Input: dimensioned drawing with shaded views. Units: mm. Origin: part minimum x, y, z. A direction names the side the tool comes from. Round coordinates to 2 decimals unless told otherwise and drop trailing zeros. Loops run counter-clockwise (first coordinate to the right, second up) from the corner with the lowest first, then second, coordinate; pieces in that order, holes last.
Item 1: Section query D-D on y = 3. Return loops of the section in (x, z) (1 decimal).
Item 2: Access query for the marked faces 5, 6, 7, 8 and 9. Directions: +Z, -Z, +X, -X, +Y, -Y. A direction counts if a zero-diameter tool reaches every point of the face in a straight line with its end or side. Return the directions, or none.
Item 3: Section query B-B on z = 23.5. Return loops of the section in (x, y) (1 decimal).
Item 4: Pull-direction query (X, two-part tool) for the marked faces 1, 2, 3 and 4; classes: released by +X, released by -X, zero draft, split by the parting line, or undercut.
Item 5: Section query C-C on x = 8. Return loops of the section in (y, z) (1 decimal), then the cut area to 3 significant figures.
Item 6: Ray query, L1, parallel to X at y = 3, z = 23.75 (1 decimal); L2, parallel to X at y = 2.25, z = 6.25; L3, parallel to Y at x = 5.75, z = 12.25. Return the intervals inside material, ascending.
Item 7: Section query A-A on x = 12. Return loops of the section in (y, z) (1 decimal).
Item 8: First-contact query: P1, Ø6, axis at x = 5, z = 3, coming from the -Y side; P2, Ø3.5, axis at y = 5, z = 10.5, coming from the +X side; P3, Ø4, axis at x = 5, y = 7.5, coming from the +Z side; P4, Ø1.3, axis at x = 4.5, y = 5.5, coming from the -Z side. Flat tips, straight axial feed; report the tip coordinate or a pass-through.
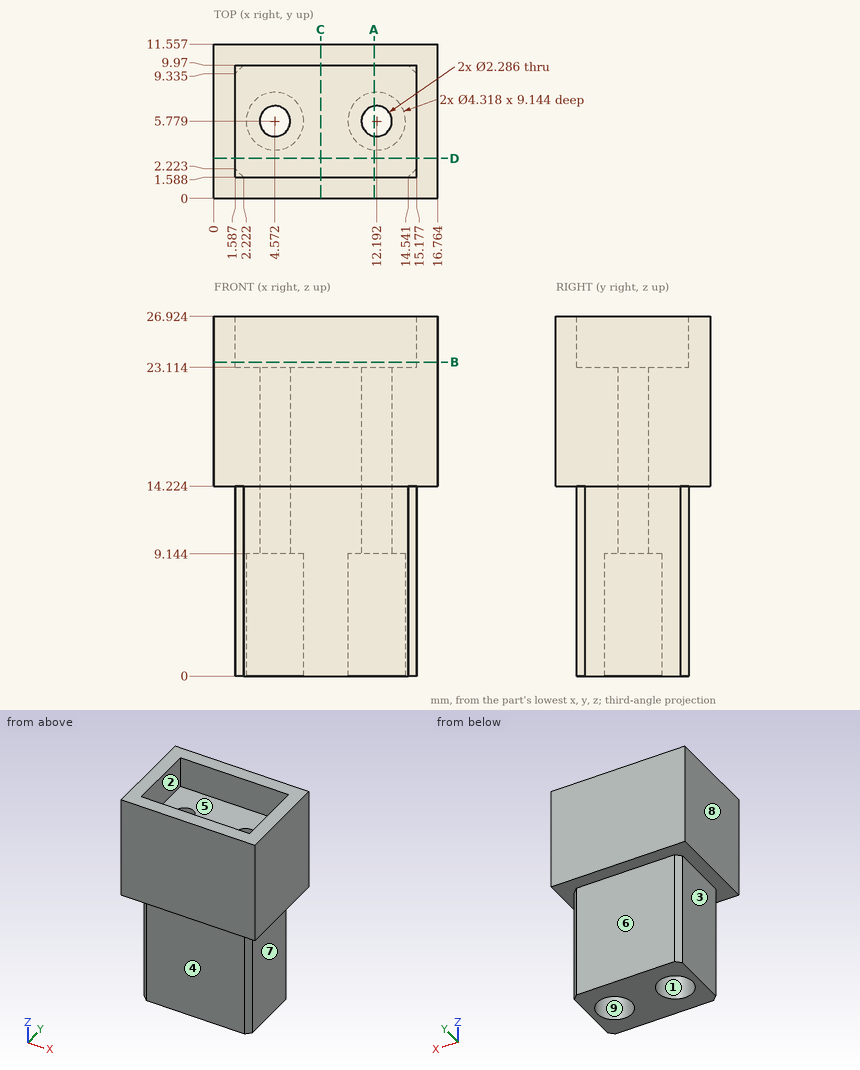
Data:
1. outline: (0, 14.2) - (1.6, 14.2) - (1.6, 0) - (15.2, 0) - (15.2, 14.2) - (16.8, 14.2) - (16.8, 26.9) - (15.2, 26.9) - (15.2, 23.1) - (1.6, 23.1) - (1.6, 26.9) - (0, 26.9) - close
2. face 5: +Z
2. face 6: -Z, +X, -X, +Y
2. face 7: -Z, +X, +Y, -Y
2. face 8: +Z, -Z, -X, +Y, -Y
2. face 9: -Z
3. outline: (0, 0) - (16.8, 0) - (16.8, 11.6) - (0, 11.6) - close; hole (1.6, 1.6) - (15.2, 1.6) - (15.2, 10) - (1.6, 10) - close
4. face 1: undercut
4. face 2: undercut
4. face 3: released by -X
4. face 4: zero draft
5. outline: (0, 14.2) - (1.6, 14.2) - (1.6, 0) - (10, 0) - (10, 14.2) - (11.6, 14.2) - (11.6, 26.9) - (10, 26.9) - (10, 23.1) - (1.6, 23.1) - (1.6, 26.9) - (0, 26.9) - close
5. area: 234 mm2
6. L1: x = 0 to 1.6, 15.2 to 16.8
6. L2: x = 1.59 to 15.18
6. L3: y = 1.59 to 9.97
7. outline: (0, 14.2) - (1.6, 14.2) - (1.6, 0) - (3.6, 0) - (3.6, 9.1) - (4.7, 9.1) - (4.7, 23.1) - (1.6, 23.1) - (1.6, 26.9) - (0, 26.9) - close; (6.9, 9.1) - (7.9, 9.1) - (7.9, 0) - (10, 0) - (10, 14.2) - (11.6, 14.2) - (11.6, 26.9) - (10, 26.9) - (10, 23.1) - (6.9, 23.1) - close
8. P1: stops at y = 1.59
8. P2: stops at x = 15.18
8. P3: stops at z = 23.11
8. P4: passes through
